Part model, mm, in its own coordinate system. Round coordinates to 2 decimals unless told otherwise and drop trailing zeros. Loops run counter-clockwise (first coordinate to the right, second up) from the corner with the lowest first, then second, coordinate; pieces in that order, holes last.
(1) Mould opens along Z. For faces 1 (the face through (0, 0, 20)), 2 (the face through (0, 0, 0)), 3 (the face through (-0.29, 2.23, 9.93)) say: +Z half, -Z half, draft (parallel to the pull), parting line (faces both ways), or undercut.
(2) Cut at C-C on z = 15.25. List the corners of the cut face in (x, y).
(3) Flat gauge pins, fed straight in: pin 1 (2.5 mm diameter, centred on x = -0.5, y = -0.5, fed in from -Z); pin 2 (3 mm diameter, centred on y = 2, z = 17, fed in from +X); pin 3 (1 mm diameter, centred on x = -1.5, z = 12, fed in from +Y); pin 4 (3 mm diameter, centred on y = -2, z = 7, fed in from -X). Where does each tip first touch, or does it go through?
(4) Cut at D-D on z = 6.5. List the corners of the cut face in (x, y), then the cut area to 3 significant figures.
(5) Probe probe 1 along Z at (x, y) = (-0.8, -2.2); probe 2 along Y at (x, z) = (0, 12.5). List the from-to ranges inside material, lowest first.
(6) Cut at A-A on y = 0. List the corners of the cut face in (x, z), then the cut area to 3 significant figures.
from build123d import *

# Parameters (mm, degrees)
SKETCH1_R           = 2.25
BOSS_EXTRUDE1_DEPTH = 20
SKETCH2_R           = 2.5
BOSS_EXTRUDE2_DEPTH = 5.3
BOSS_EXTRUDE3_START = -14.7
SKETCH2_2_R         = 2.5
BOSS_EXTRUDE3_DEPTH = 5.3


with BuildPart() as part:
    # Sketch1 → Boss-Extrude1 (new body)
    with BuildSketch(Plane.XY):
        Circle(SKETCH1_R)
    extrude(amount=BOSS_EXTRUDE1_DEPTH)

    # Sketch2 → Boss-Extrude2 (add)
    with BuildSketch(Plane(origin=(0, 0, 0), x_dir=(-1, 0, 0), z_dir=(0, 0, -1))):
        Circle(SKETCH2_R)
    extrude(amount=-BOSS_EXTRUDE2_DEPTH)

    # Sketch2<2> → Boss-Extrude3 (add)
    with BuildSketch(Plane(origin=(0, 0, 0), x_dir=(-1, 0, 0), z_dir=(0, 0, -1)).offset(BOSS_EXTRUDE3_START)):
        Circle(SKETCH2_2_R)
    extrude(amount=-BOSS_EXTRUDE3_DEPTH)


solid = part.part
Final values:
1. face 1: +Z half
1. face 2: -Z half
1. face 3: undercut
2. outline: circle Ø5 at (0, 0)
3. pin 1: stops at z = 0
3. pin 2: stops at x = 2.45
3. pin 3: stops at y = 2.02
3. pin 4: stops at x = -2.19
4. outline: circle Ø4.5 at (0, 0)
4. area: 15.9 mm2
5. probe 1: z = 0 to 5.3, 14.7 to 20
5. probe 2: y = -2.25 to 2.25
6. outline: (-2.5, 0) - (2.5, 0) - (2.5, 5.3) - (2.25, 5.3) - (2.25, 14.7) - (2.5, 14.7) - (2.5, 20) - (-2.5, 20) - (-2.5, 14.7) - (-2.25, 14.7) - (-2.25, 5.3) - (-2.5, 5.3) - close
6. area: 95.3 mm2
